```python
from build123d import *

# Parameters (mm, degrees)
BOSS_EXTRUDE1_DEPTH        = 42
CUT_EXTRUDE1_DEPTH         = 43
CUT_EXTRUDE2_DEPTH         = 43
CUT_EXTRUDE3_DEPTH         = 43
SKETCH10_W                 = 42
SKETCH10_H                 = 2.075
SKETCH11_W                 = 42
SKETCH11_H                 = 2.075
SKETCH12_W                 = 42
SKETCH12_H                 = 2.075
M3_5_CLEARANCE_HOLE1_D     = 4.134
M3_5_CLEARANCE_HOLE1_DEPTH = 5
M3_5_CLEARANCE_HOLE1_TIP   = 1.193383006
CHAMFER1_SIZE              = 0.379


with BuildPart() as part:
    # Sketch1 → Boss-Extrude1 (new body)
    with BuildSketch(Plane(origin=(42, 0, 0), x_dir=(0, 0, -1), z_dir=(1, 0, 0))):
        with BuildLine():
            Line((-12.5, 9.987492178), (-12.5, -9.987492178))
            ThreePointArc((-12.5, -9.987492178), (-11.313708499, -11.313708499), (-9.987492178, -12.5))
            Line((-9.987492178, -12.5), (9.987492178, -12.5))
            ThreePointArc((9.987492178, -12.5), (11.313708499, -11.313708499), (12.5, -9.987492178))
            Line((12.5, -9.987492178), (12.5, 9.987492178))
            ThreePointArc((12.5, 9.987492178), (11.313708499, 11.313708499), (9.987492178, 12.5))
            Line((9.987492178, 12.5), (-9.987492178, 12.5))
            ThreePointArc((-9.987492178, 12.5), (-11.313708499, 11.313708499), (-12.5, 9.987492178))
        make_face()
    extrude(amount=-BOSS_EXTRUDE1_DEPTH)

    # Sketch2 → Cut-Extrude1 (cut, through all)
    with BuildSketch(Plane.ZY):
        with BuildLine():
            Line((12.5, -1.5), (12.5, 1.5))
            Line((12.5, 1.5), (10.933745096, 1.5))
            ThreePointArc((10.933745096, 1.5), (11.575, 0), (10.933745096, -1.5))
            Line((10.933745096, -1.5), (12.5, -1.5))
        make_face()
    extrude(amount=-CUT_EXTRUDE1_DEPTH, mode=Mode.SUBTRACT)

    # Sketch3 → Cut-Extrude2 (cut, through all)
    with BuildSketch(Plane.ZY):
        with BuildLine():
            Line((-1.5, -12.5), (1.5, -12.5))
            Line((1.5, -12.5), (1.5, -10.933745096))
            ThreePointArc((1.5, -10.933745096), (0, -11.575), (-1.5, -10.933745096))
            Line((-1.5, -10.933745096), (-1.5, -12.5))
        make_face()
    extrude(amount=-CUT_EXTRUDE2_DEPTH, mode=Mode.SUBTRACT)

    # Sketch4 → Cut-Extrude3 (cut, through all)
    with BuildSketch(Plane.ZY):
        with BuildLine():
            Line((-12.5, 1.5), (-12.5, -1.5))
            Line((-12.5, -1.5), (-10.933745096, -1.5))
            ThreePointArc((-10.933745096, -1.5), (-11.575, 0), (-10.933745096, 1.5))
            Line((-10.933745096, 1.5), (-12.5, 1.5))
        make_face()
    extrude(amount=-CUT_EXTRUDE3_DEPTH, mode=Mode.SUBTRACT)

    # Sketch5 → Cut-Revolve1 (revolve, cut)
    with BuildSketch(Plane.XY):
        Polygon((0, 6.5), (0, 0), (36, 0), (36, 6), (11, 6), (11, 3), (1.2, 3), (1.2, 6.5), align=None)
    revolve(axis=Axis((0, 0, 0), (1, 0, 0)), mode=Mode.SUBTRACT)

    # Sketch6 → Cut-Revolve2 (revolve, cut)
    with BuildSketch(Plane(origin=(0, 0, -7.75), x_dir=(-1, 0, 0), z_dir=(0, 0, -1))):
        Polygon((-42, 11), (-42, 7.75), (0, 7.75), (0, 11), (-4, 11), (-4, 9.371), (-11, 9.371), (-11.074478185, 9.5), (-30.925521815, 9.5), (-31, 9.371), (-38, 9.371), (-38, 11), align=None)
    revolve(axis=Axis((42, 7.75, -7.75), (-1, 0, 0)), mode=Mode.SUBTRACT)

    # Sketch7 → Cut-Revolve3 (revolve, cut)
    with BuildSketch(Plane(origin=(0, 0, -7.75), x_dir=(-1, 0, 0), z_dir=(0, 0, -1))):
        Polygon((-42, -4.5), (-42, -7.75), (0, -7.75), (0, -4.5), (-4, -4.5), (-4, -6.129), (-11, -6.129), (-11.074478185, -6), (-30.925521815, -6), (-31, -6.129), (-38, -6.129), (-38, -4.5), align=None)
    revolve(axis=Axis((42, -7.75, -7.75), (-1, 0, 0)), mode=Mode.SUBTRACT)

    # Sketch8 → Cut-Revolve4 (revolve, cut)
    with BuildSketch(Plane(origin=(0, 0, 7.75), x_dir=(-1, 0, 0), z_dir=(0, 0, -1))):
        Polygon((-42, -4.5), (-42, -7.75), (0, -7.75), (0, -4.5), (-4, -4.5), (-4, -6.129), (-11, -6.129), (-11.074478185, -6), (-30.925521815, -6), (-31, -6.129), (-38, -6.129), (-38, -4.5), align=None)
    revolve(axis=Axis((42, -7.75, 7.75), (-1, 0, 0)), mode=Mode.SUBTRACT)

    # Sketch9 → Cut-Revolve5 (revolve, cut)
    with BuildSketch(Plane(origin=(0, 0, 7.75), x_dir=(-1, 0, 0), z_dir=(0, 0, -1))):
        Polygon((-42, 11), (-42, 7.75), (0, 7.75), (0, 11), (-4, 11), (-4, 9.371), (-11, 9.371), (-11.074478185, 9.5), (-30.925521815, 9.5), (-31, 9.371), (-38, 9.371), (-38, 11), align=None)
    revolve(axis=Axis((42, 7.75, 7.75), (-1, 0, 0)), mode=Mode.SUBTRACT)

    # Sketch10 → Cut-Revolve6 (revolve, cut)
    with BuildSketch(Plane.XY.offset(9.5)):
        with Locations((21, 1.0375)):
            Rectangle(SKETCH10_W, SKETCH10_H)
    revolve(axis=Axis((0, 0, 9.5), (1, 0, 0)), mode=Mode.SUBTRACT)

    # Sketch11 → Cut-Revolve7 (revolve, cut)
    with BuildSketch(Plane.XY):
        with Locations((21, -8.4625)):
            Rectangle(SKETCH11_W, SKETCH11_H)
    revolve(axis=Axis((0, -9.5, 0), (1, 0, 0)), mode=Mode.SUBTRACT)

    # Sketch12 → Cut-Revolve8 (revolve, cut)
    with BuildSketch(Plane.XY.offset(-9.5)):
        with Locations((21, 1.0375)):
            Rectangle(SKETCH12_W, SKETCH12_H)
    revolve(axis=Axis((0, 0, -9.5), (1, 0, 0)), mode=Mode.SUBTRACT)

    # M3.5 Clearance Hole1
    with Locations(Plane(origin=(0, 12.5, 0), x_dir=(1, 0, 0), z_dir=(0, 1, 0))):
        with Locations((7.5, 0), (37, 0)):
            Hole(M3_5_CLEARANCE_HOLE1_D / 2, depth=M3_5_CLEARANCE_HOLE1_DEPTH)
            with Locations((0, 0, -(M3_5_CLEARANCE_HOLE1_DEPTH + M3_5_CLEARANCE_HOLE1_TIP / 2))):  # 120° drill point
                Cone(0, M3_5_CLEARANCE_HOLE1_D / 2, M3_5_CLEARANCE_HOLE1_TIP, mode=Mode.SUBTRACT)

    # Chamfer1
    chamfer1_edges = [part.edges().sort_by_distance(p)[0] for p in [
        (4, -9.371, 7.75),
        (38, -9.371, 7.75),
        (4, 6.129, 7.75),
        (38, 6.129, 7.75),
        (39.067, 12.5, 0),
        (9.567, 12.5, 0),
        (4, 6.129, -7.75),
        (38, 6.129, -7.75),
        (4, -9.371, -7.75),
        (38, -9.371, -7.75),
    ]]
    chamfer(chamfer1_edges, length=CHAMFER1_SIZE)


solid = part.part
```
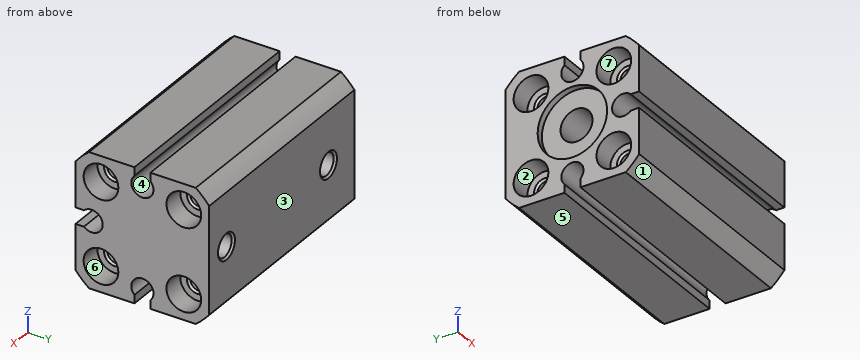
The listing builds one solid part. Answer for the finished solid, in the listing's coordinates (mm). Face numbers are marked on the shaded views. A direction names the side the tool comes from. Give positions to 0.01 mm unless a question says otherwise; leave off trailing zeros. Use one line per item in the form item = value. Start each with the question number.
1) The mould has two halves that part along Z. Classify the marked faces 1, 2, 3 and 4: pulls with the +Z half, pulls with the -Z half, needs draft (parallel to the pull), parting line crosses it, or undercut.
2) Flat-ended cylindrical pins translate along their axes: pin 1 Ø4 at (y, z) = (6, 2) entering from -X; pin 2 Ø1.9 at (y, z) = (-7.75, -7.75) entering from -X; pin 3 Ø3.5 at (y, z) = (7.75, 7.75) entering from +X; pin 4 Ø1.7 at (x, y) = (11, -12) entering from +Z. Find the tip coordinate at first contact, or state that the pin passes through.
3) Consider line 1 along Z through (x, y) = (2.7, 7.75); line 2 along Z through (x, y) = (25, 7.75); line 3 along Z through (x, y) = (7.5, -8). Determine where each line is inside the solid, lowest interval first. Write a range as from..to.
4) Find section A-A on x = 31.5. Count the separate pieces of the cut face and the enclosed holes in it, plus the area to 3 significant figures.
5) A tool of negligible diameter and unlimited length cuts with its end or side. For the marked faces 5, 6 and 7, from which of +Z, -Z, +X, -X, +Y, -Y can it reach the whole face along a straight path? Write none if from no direction.
Geometry results:
q1.face_1 = pulls with the -Z half
q1.face_2 = undercut
q1.face_3 = needs draft
q1.face_4 = undercut
q2.pin_1 = 0
q2.pin_2 = through
q2.pin_3 = 37.75
q2.pin_4 = 11.48
q3.line_1 = -12.5..-11, -4.5..4.5, 11..12.5
q3.line_2 = -12.5..-9.5, -6..6, 9.5..12.5
q3.line_3 = -12.5..-9.35, -6.15..-1.43, 1.43..6.15, 9.35..12.5
q4.separate_pieces = 1
q4.enclosed_holes = 5
q4.area = 417 mm2
q5.face_5 = -Z, +X, -X, +Y, -Y
q5.face_6 = +X
q5.face_7 = -X
